Build history of the part. All positions in model axes, mm. Face numbers are marked on the shaded views. A direction names the side the tool comes from. Coordinates: 2 decimals unless noted, no trailing zeros. Loops run counter-clockwise (first coordinate to the right, second up) from the corner with the lowest first, then second, coordinate; pieces in that order, holes last.
Item 1: Cut at C-C (x = 137). List the corners of the cut face in (y, z), and give its area (3 significant figures).
Item 2: Drill centre lines: line 1 along Y through (x, z) = (121.5, 7.5); line 2 along X through (y, z) = (45, 13.5). Where is each one in solid material? Low to high.
Item 3: Cut at D-D (z = 41). List the corners of the cut face in (x, y).
Item 4: Cut at B-B (y = 10.5). List the corners of the cut face in (x, z), and give its area (3 significant figures).
Item 5: Cut at A-A (z = 12.5). List the corners of the cut face in (x, y), and give its area (3 significant figures).
Item 6: 3-axis set-ups, long thin cutter, end or side, ignore diameter. For the marked faces 1, 2 and 3: which of +Z, -Z, +X, -X, +Y, -Y reach the whole face in a straight line?
Item 7: Flat gauge pins, fed straight in: pin 1 (15 mm diameter, centred on x = 120.5, z = 24, fed in from -Y); pin 2 (20.5 mm diameter, centred on x = 124, y = 68, fed in from +Z); pin 3 (6 mm diameter, centred on y = 42, z = 24.5, fed in from +X). Where does each tip first touch, or does it go through?
from build123d import *

# Parameters (mm, degrees)
F0_W     = 152.4
F0_H     = 50.8
F1_DEPTH = 76.2
F2_W     = 127
F2_H     = 50.8
F3_DEPTH = 50.8
F4_W     = 50.8
F4_H     = 25.4
F5_DEPTH = 76.2


with BuildPart() as f1:
    # F0 (on Front) → F1 (new body)
    with BuildSketch(Plane.XZ):
        with Locations((76.2, 25.4)):
            Rectangle(F0_W, F0_H)
    extrude(amount=-F1_DEPTH)

    # F2 (on Front) → F3 (cut)
    with BuildSketch(Plane.XZ):
        with Locations((88.9, 25.4)):
            Rectangle(F2_W, F2_H)
    extrude(amount=-F3_DEPTH, mode=Mode.SUBTRACT)

    # F4 (on Front) → F5 (cut)
    with BuildSketch(Plane.XZ):
        with Locations((127, 38.1)):
            Rectangle(F4_W, F4_H)
    extrude(amount=-F5_DEPTH, mode=Mode.SUBTRACT)


solid = f1.part
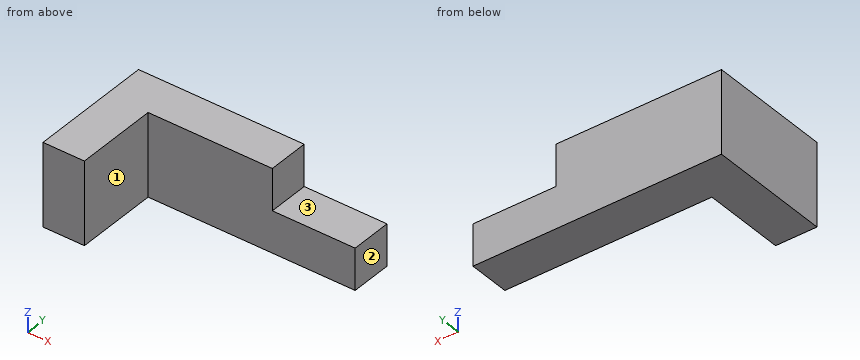
Filled sheet:
1. outline: (50.8, 0) - (76.2, 0) - (76.2, 25.4) - (50.8, 25.4) - close
1. area: 645 mm2
2. line 1: y = 50.8 to 76.2
2. line 2: x = 0 to 25.4
3. outline: (0, 0) - (25.4, 0) - (25.4, 50.8) - (101.6, 50.8) - (101.6, 76.2) - (0, 76.2) - close
4. outline: (0, 0) - (25.4, 0) - (25.4, 50.8) - (0, 50.8) - close
4. area: 1,290 mm2
5. outline: (0, 0) - (25.4, 0) - (25.4, 50.8) - (152.4, 50.8) - (152.4, 76.2) - (0, 76.2) - close
5. area: 5,160 mm2
6. face 1: +Z, -Z, +X, -Y
6. face 2: +Z, -Z, +X, +Y, -Y
6. face 3: +Z, +X, +Y, -Y
7. pin 1: stops at y = 50.8
7. pin 2: stops at z = 25.4
7. pin 3: stops at x = 25.4
